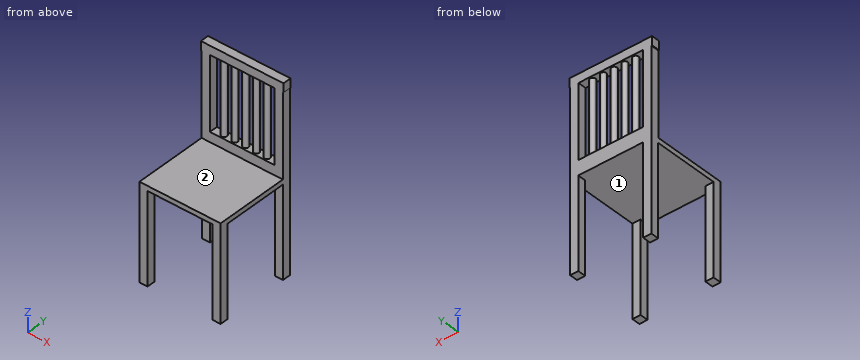
```python
from build123d import *

# Parameters (mm, degrees)
F0_W      = 83
F0_H      = 83
F1_DEPTH  = 5
F2_W      = 83
F2_H      = 8.5
F3_DEPTH  = 10
F4_W      = 8.5
F4_H      = 8.5
F5_DEPTH  = 75
F6_R      = 2.85
F7_DEPTH  = 75
F8_W      = 83
F8_H      = 8.5
F8_R      = 2.85
F8_W_2    = 0.7
F9_DEPTH  = 9
F10_W     = 8.3
F10_H     = 8.3
F11_DEPTH = 93


with BuildPart() as f1:
    # F0 (on Top) → F1 (new body)
    with BuildSketch(Plane.XY):
        Rectangle(F0_W, F0_H)
    extrude(amount=F1_DEPTH)

    # F2 (on face) → F3 (join)
    with BuildSketch(Plane.XY.offset(5)):
        with Locations((0, 37.25)):
            Rectangle(F2_W, F2_H)
    extrude(amount=F3_DEPTH)

    # F4 (on face) → F5 (join)
    with BuildSketch(Plane.XY.offset(15)):
        with Locations((-37.25, 37.25)):
            Rectangle(F4_W, F4_H)
        with Locations((37.25, 37.25)):
            Rectangle(F4_W, F4_H)
    extrude(amount=F5_DEPTH)

    # F6 (on face) → F7 (join)
    with BuildSketch(Plane.XY.offset(15)):
        with Locations((-21.999383, 37.25)):
            Circle(F6_R)
        with Locations((-10.916319, 37.250001)):
            Circle(F6_R)
        with Locations((0, 37.25)):
            Circle(F6_R)
        with Locations((10.916319, 37.250001)):
            Circle(F6_R)
        with Locations((21.999383, 37.25)):
            Circle(F6_R)
    extrude(amount=F7_DEPTH)

    # F8 (on face) → F9 (join)
    with BuildSketch(Plane.XY.offset(90)):
        with Locations((0, 37.25)):
            Rectangle(F8_W, F8_H)
        with Locations((0, 37.25)):
            Circle(F8_R, mode=Mode.SUBTRACT)
        with Locations((0, 37.25)):
            Circle(F8_R)
        with Locations((-41.85, 37.25)):
            Rectangle(F8_W_2, F8_H)
        with Locations((41.85, 37.25)):
            Rectangle(F8_W_2, F8_H)
    extrude(amount=F9_DEPTH)

    # F10 (on face) → F11 (join)
    with BuildSketch(Plane(origin=(0, 0, 0), x_dir=(1, 0, 0), z_dir=(0, 0, -1))):
        with Locations((-37.35, 37.35)):
            Rectangle(F10_W, F10_H)
        with Locations((37.35, 37.35)):
            Rectangle(F10_W, F10_H)
        with Locations((-37.35, -37.35)):
            Rectangle(F10_W, F10_H)
        with Locations((37.35, -37.35)):
            Rectangle(F10_W, F10_H)
    extrude(amount=F11_DEPTH)


solid = f1.part
```
Source: CAD feature listing. Evaluate the final solid. Frame: model axes, mm. Face numbers are marked on the shaded views. Coordinates: 2 decimals unless noted, no trailing zeros. Order: outer loops, then holes, each group sorted by start corner. A loop starts at its lowest first (then second) coordinate and runs counter-clockwise, first axis right, second up. Notation, with made-up numbers: (62, 64) - (83, 64) arc R27 cw to (83, 81) - close; hole circle Ø6 at (16.5, 52.5). An arc over 180 degrees is marked (long way). One line per item, written item: value.
1) Mould query, pull axis X, two halves, no side actions, for the marked faces 1 and 2. Classes: released by +X, released by -X, zero draft, split by the parting line, or undercut.
Computed values:
face 1: undercut
face 2: zero draft
2) Cut plane D-D on z = 12.5. Output: boundary loops of the cut face in (x, y).
Computed values:
outline: (-41.5, 33) - (41.5, 33) - (41.5, 41.5) - (-41.5, 41.5) - close
3) Cut plane C-C on y = 37.25. State how many separate pieces and enclosed holes the cut face has, plus the area to 3 significant figures.
Computed values:
separate pieces: 1
enclosed holes: 6
area: 6,960 mm^2
4) Cut plane A-A on z = 86. Output: boundary loops of the cut face in (x, y).
Computed values:
outline: (-41.5, 33) - (-33, 33) - (-33, 41.5) - (-41.5, 41.5) - close; circle Ø5.7 at (-22, 37.25); circle Ø5.7 at (-10.92, 37.25); circle Ø5.7 at (0, 37.25); circle Ø5.7 at (10.92, 37.25); circle Ø5.7 at (22, 37.25); (33, 33) - (41.5, 33) - (41.5, 41.5) - (33, 41.5) - close
5) Cut plane B-B on x = 6. Output: boundary loops of the cut face in (y, z), plus the area to 4 significant figures.
Computed values:
outline: (-41.5, 0) - (41.5, 0) - (41.5, 15) - (33, 15) - (33, 5) - (-41.5, 5) - close; (33, 90) - (41.5, 90) - (41.5, 99) - (33, 99) - close
area: 576.5 mm^2
6) Contact query for flat-ended pins moving along their axis: pin 1 (8 mm diameter, centred on x = 24.5, z = 47.5, fed in from +Y); pin 2 (2.5 mm diameter, centred on y = -38.5, z = -68.5, fed in from -X); pin 3 (6 mm diameter, centred on x = -6, z = 77.5, fed in from +Y). Output: stop coordinate, or through.
Computed values:
pin 1: stops at y = 40.1
pin 2: stops at x = -41.5
pin 3: stops at y = 39.36
7) Ray query, line 1 (Y direction, x = 38, z = -20.5); line 2 (X direction, y = 34, z = 86); line 3 (Z direction, x = -4, y = -33). Return the intervals inside material, ascending. Write a range as [from, to].
Computed values:
line 1: y = [-41.5, -33.2], [33.2, 41.5]
line 2: x = [-41.5, -33], [33, 41.5]
line 3: z = [0, 5]
